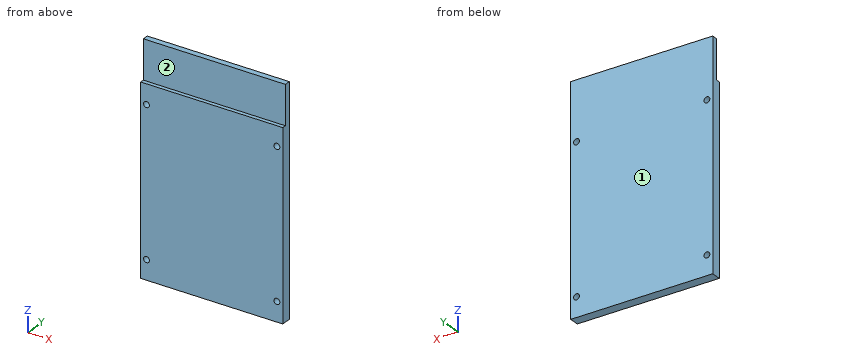
Autodesk Inventor part; units mm, degrees
ref_plane "YZ Plane" through (0, 0, 0) normal (1, 0, 0) x (0, 1, 0)
ref_plane "XZ Plane" through (0, 0, 0) normal (0, 1, 0) x (-1, 0, 0)
ref_plane "XY Plane" through (0, 0, 0) normal (0, 0, 1) x (1, 0, 0)
sketch "Sketch1" plane through (0, 0, 0) normal (0, 1, 0) x (-1, 0, 0)
  line L0 (0, 0) -> (-73, 0)
  line L1 (-73, 0) -> (-73, -115)
  line L2 (-73, -115) -> (0, -115)
  line L3 (0, -115) -> (0, 0)
  dimension "d0" = 115
  dimension "d1" = 73
extrude "Extrusion1" add sketch "Sketch1" along normal blind 5
sketch "Sketch2" plane through (73, 0, 0) normal (1, 0, 0) x (0, 0, -1)
  line L0 (0, 0) -> (0, 5) construction
  line L1 (0, 0) -> (115, 0) construction
  line L2 (0, 2) -> (20, 2)
  line L3 (20, 2) -> (20, 0)
  line L4 (0, 2) -> (0, 0)
  line L5 (20, 0) -> (0, 0)
  dimension "d4" = 20
  dimension "d5" = 2
extrude "Extrusion2" cut sketch "Sketch2" against normal through all
sketch "Sketch3" plane through (0, 0, 0) normal (0, -1, 0) x (1, 0, 0)
  line L0 (0, -115) -> (0, 0) construction
  line L1 (73, -115) -> (0, -115) construction
  line L2 (0, 0) -> (73, 0) construction
  line L3 (73, 0) -> (73, -115) construction
  line L4 (73, -20) -> (0, -20) construction
  line L5 (36.5, -115) -> (36.5, -20) construction
  line L6 (73, -20) -> (0, -20) construction
  point P0 (3, -105)
  point P1 (3, -30)
  point P2 (70, -105)
  point P3 (70, -30)
  dimension "d8" = 10
  dimension "d9" = 3
  dimension "d10" = 3
  dimension "d11" = 10
hole "Hole1" at (3, 0, -105) at (3, 0, -30) at (70, 0, -105) at (70, 0, -30) direction (0, 1, 0) diameter 3 end through all
properties part number "arduinoShelf" material "Plywood, Sheathing"
Build history of the part. All positions in model axes, mm. Face numbers are marked on the shaded views. A direction names the side the tool comes from. Coordinates: 2 decimals unless noted, no trailing zeros. Order: outer loops, then holes, each group sorted by start corner. A loop starts at its lowest first (then second) coordinate and runs counter-clockwise, first axis right, second up. Notation, with made-up numbers: (8.5, 61.25) - (18.5, 61.25) arc R28 cw to (18.5, 99.25) - close; hole circle Ø5 at (18.25, 15). An arc over 180 degrees is marked (long way). Put each result on its own line as item: value.
1. Saw through at B-B (z = -105). Write the cut outline in (x, y), and give its area (3 significant figures).
Answer sheet:
outline: (0, 0) - (1.5, 0) - (1.5, 5) - (0, 5) - close; (4.5, 0) - (68.5, 0) - (68.5, 5) - (4.5, 5) - close; (71.5, 0) - (73, 0) - (73, 5) - (71.5, 5) - close
area: 335 mm^2
2. Saw through at A-A (x = 70). Write the cut outline in (y, z), and give its area (3 significant figures).
Answer sheet:
outline: (0, -115) - (5, -115) - (5, -106.5) - (0, -106.5) - close; (0, -103.5) - (5, -103.5) - (5, -31.5) - (0, -31.5) - close; (0, -28.5) - (5, -28.5) - (5, 0) - (2, 0) - (2, -20) - (0, -20) - close
area: 505 mm^2
3. Tool access for the marked faces 1 and 2: list every direction of +Z, -Z, +X, -X, +Y, -Y with a clear straight run to the whole face (end or side of a thin tool).
Answer sheet:
face 1: +Z, -Z, +X, -X, +Y
face 2: +Z, +X, -X, -Y
4. Drop flat-ended pins along their axis: P1, Ø1, axis at x = 42.5, y = 1, coming from the +Z side; P2, Ø1, axis at x = 29.5, z = -14.5, coming from the -Y side. Give the stop position or say it passes through.
Answer sheet:
P1: stops at z = -20
P2: stops at y = 2
5. Probe line 1 along Z through (x, y) = (70, 3.75); line 2 along X through (y, z) = (3.8, -30); line 3 along Z through (x, y) = (33.5, 0.9). List the from-to ranges inside material, lowest first. Write a range as [from, to].
Answer sheet:
line 1: z = [-115, -106.5], [-103.5, -31.5], [-28.5, 0]
line 2: x = [0, 1.5], [4.5, 68.5], [71.5, 73]
line 3: z = [-115, -20]
